from build123d import *

# Parameters (mm, degrees)
ESQUISSE1_R                            = 1.5
BOSS_EXTRU_1_DEPTH                     = 4
ESQUISSE2_R                            = 3.25
BOSS_EXTRU_2_DEPTH                     = 4
BOSS_EXTRU_3_START                     = -1
BOSS_EXTRU_3_DEPTH                     = 1
R_P_TITION_CIRCULAIRE6_COUNT           = 4
ESQUISSE5_R                            = 0.5
ENL_V_MAT_EXTRU_1_DEPTH                = 1
R_P_TITION_LIN_AIRE1_COUNT             = 3
R_P_TITION_LIN_AIRE1_PITCH             = 2
R_P_TITION_CIRCULAIRE7_COUNT           = 4
R_P_TITION_CIRCULAIRE7_COPY_1_SKETCH_R = 0.5
R_P_TITION_CIRCULAIRE7_COPY_1_DEPTH    = 1
R_P_TITION_CIRCULAIRE7_COPY_2_SKETCH_R = 0.5
R_P_TITION_CIRCULAIRE7_COPY_2_DEPTH    = 1
R_P_TITION_CIRCULAIRE7_COPY_3_SKETCH_R = 0.5
R_P_TITION_CIRCULAIRE7_COPY_3_DEPTH    = 1
R_P_TITION_CIRCULAIRE7_COPY_4_SKETCH_R = 0.5
R_P_TITION_CIRCULAIRE7_COPY_4_DEPTH    = 1
R_P_TITION_CIRCULAIRE7_COPY_5_SKETCH_R = 0.5
R_P_TITION_CIRCULAIRE7_COPY_5_DEPTH    = 1
R_P_TITION_CIRCULAIRE7_COPY_6_SKETCH_R = 0.5
R_P_TITION_CIRCULAIRE7_COPY_6_DEPTH    = 1
ESQUISSE6_R                            = 2.5
ENL_V_MAT_EXTRU_2_DEPTH                = 1
ESQUISSE7_R                            = 0.75
ENL_V_MAT_EXTRU_3_DEPTH                = 2


with BuildPart() as part:
    # Esquisse1 → Boss.-Extru.1 (new body)
    with BuildSketch(Plane(origin=(0, 0, 0), x_dir=(1, 0, 0), z_dir=(0, 1, 0))):
        with Locations(Location((0, 0, 0), (0, 0, 270))):
            Circle(ESQUISSE1_R)
    extrude(amount=BOSS_EXTRU_1_DEPTH)

    # Esquisse2 → Boss.-Extru.2 (add)
    with BuildSketch(Plane(origin=(0, 4, 0), x_dir=(1, 0, 0), z_dir=(0, 1, 0))):
        with Locations(Location((0, 0, 0), (0, 0, 270))):
            Circle(ESQUISSE2_R)
    extrude(amount=BOSS_EXTRU_2_DEPTH)

    # Esquisse3 → Boss.-Extru.3 (add)
    with BuildSketch(Plane(origin=(0, 8, 0), x_dir=(1, 0, 0), z_dir=(0, 1, 0)).offset(BOSS_EXTRU_3_START)):
        with BuildLine():
            ThreePointArc((-2, -8.5), (-1.25, -9.583333333), (0, -10))
            ThreePointArc((0, -10), (1.25, -9.583333333), (2, -8.5))
            Line((2, -8.5), (2, -2.561737691))
            ThreePointArc((2, -2.561737691), (0, -3.25), (-2, -2.561737691))
            Line((-2, -2.561737691), (-2, -8.5))
        make_face()
    boss_extru_3 = extrude(amount=BOSS_EXTRU_3_DEPTH)

    # Répétition circulaire6: Boss.-Extru.3 ×4 about axis
    r_p_tition_circulaire6_axis = Axis((0, 0, 0), (0, 1, 0))
    for i in range(1, R_P_TITION_CIRCULAIRE6_COUNT):
        add(boss_extru_3.rotate(r_p_tition_circulaire6_axis, i * 360 / R_P_TITION_CIRCULAIRE6_COUNT))

    # Esquisse5 → Enlèv. mat.-Extru.1 (cut)
    with BuildSketch(Plane(origin=(0, 8, 0), x_dir=(1, 0, 0), z_dir=(0, 1, 0))):
        with Locations(Location((0, -8.5, 0), (0, 0, 270))):
            Circle(ESQUISSE5_R)
    enl_v_mat_extru_1 = extrude(amount=-ENL_V_MAT_EXTRU_1_DEPTH, mode=Mode.SUBTRACT)

    # Répétition linéaire1: Enlèv. mat.-Extru.1 ×3
    with Locations(*[(0, 0, -i * R_P_TITION_LIN_AIRE1_PITCH) for i in range(1, R_P_TITION_LIN_AIRE1_COUNT)]):
        add(enl_v_mat_extru_1, mode=Mode.SUBTRACT)

    # Répétition circulaire7: Enlèv. mat.-Extru.1 ×4 about axis
    r_p_tition_circulaire7_axis = Axis((0, 0, 0), (0, 1, 0))
    for i in range(1, R_P_TITION_CIRCULAIRE7_COUNT):
        add(enl_v_mat_extru_1.rotate(r_p_tition_circulaire7_axis, i * 360 / R_P_TITION_CIRCULAIRE7_COUNT), mode=Mode.SUBTRACT)

    # Répétition circulaire7 copy 1 sketch → Répétition circulaire7 copy 1 (cut)
    with BuildSketch(Plane(origin=(-2, 8, 0), x_dir=(0, 0, -1), z_dir=(0, 1, 0))):
        with Locations(Location((0, -8.5, 0), (0, 0, 270))):
            Circle(R_P_TITION_CIRCULAIRE7_COPY_1_SKETCH_R)
    extrude(amount=-R_P_TITION_CIRCULAIRE7_COPY_1_DEPTH, mode=Mode.SUBTRACT)

    # Répétition circulaire7 copy 2 sketch → Répétition circulaire7 copy 2 (cut)
    with BuildSketch(Plane(origin=(0, 8, 2), x_dir=(-1, 0, 0), z_dir=(0, 1, 0))):
        with Locations(Location((0, -8.5, 0), (0, 0, 270))):
            Circle(R_P_TITION_CIRCULAIRE7_COPY_2_SKETCH_R)
    extrude(amount=-R_P_TITION_CIRCULAIRE7_COPY_2_DEPTH, mode=Mode.SUBTRACT)

    # Répétition circulaire7 copy 3 sketch → Répétition circulaire7 copy 3 (cut)
    with BuildSketch(Plane(origin=(2, 8, 0), x_dir=(0, 0, 1), z_dir=(0, 1, 0))):
        with Locations(Location((0, -8.5, 0), (0, 0, 270))):
            Circle(R_P_TITION_CIRCULAIRE7_COPY_3_SKETCH_R)
    extrude(amount=-R_P_TITION_CIRCULAIRE7_COPY_3_DEPTH, mode=Mode.SUBTRACT)

    # Répétition circulaire7 copy 4 sketch → Répétition circulaire7 copy 4 (cut)
    with BuildSketch(Plane(origin=(-4, 8, 0), x_dir=(0, 0, -1), z_dir=(0, 1, 0))):
        with Locations(Location((0, -8.5, 0), (0, 0, 270))):
            Circle(R_P_TITION_CIRCULAIRE7_COPY_4_SKETCH_R)
    extrude(amount=-R_P_TITION_CIRCULAIRE7_COPY_4_DEPTH, mode=Mode.SUBTRACT)

    # Répétition circulaire7 copy 5 sketch → Répétition circulaire7 copy 5 (cut)
    with BuildSketch(Plane(origin=(0, 8, 4), x_dir=(-1, 0, 0), z_dir=(0, 1, 0))):
        with Locations(Location((0, -8.5, 0), (0, 0, 270))):
            Circle(R_P_TITION_CIRCULAIRE7_COPY_5_SKETCH_R)
    extrude(amount=-R_P_TITION_CIRCULAIRE7_COPY_5_DEPTH, mode=Mode.SUBTRACT)

    # Répétition circulaire7 copy 6 sketch → Répétition circulaire7 copy 6 (cut)
    with BuildSketch(Plane(origin=(4, 8, 0), x_dir=(0, 0, 1), z_dir=(0, 1, 0))):
        with Locations(Location((0, -8.5, 0), (0, 0, 270))):
            Circle(R_P_TITION_CIRCULAIRE7_COPY_6_SKETCH_R)
    extrude(amount=-R_P_TITION_CIRCULAIRE7_COPY_6_DEPTH, mode=Mode.SUBTRACT)

    # Esquisse6 → Enlèv. mat.-Extru.2 (cut)
    with BuildSketch(Plane(origin=(0, 8, 0), x_dir=(1, 0, 0), z_dir=(0, 1, 0))):
        with Locations(Location((0, 0, 0), (0, 0, 270))):
            Circle(ESQUISSE6_R)
    extrude(amount=-ENL_V_MAT_EXTRU_2_DEPTH, mode=Mode.SUBTRACT)

    # Esquisse7 → Enlèv. mat.-Extru.3 (cut)
    with BuildSketch(Plane(origin=(0, 7, 0), x_dir=(1, 0, 0), z_dir=(0, 1, 0))):
        with Locations(Location((0, 0, 0), (0, 0, 270))):
            Circle(ESQUISSE7_R)
    extrude(amount=-ENL_V_MAT_EXTRU_3_DEPTH, mode=Mode.SUBTRACT)


solid = part.part
Here's how the part is built. I have some questions about the finished solid (model axes, mm). A direction names the side the tool comes from. Coordinates: 2 decimals unless noted, no trailing zeros. Write each loop counter-clockwise with the first axis right and the second up, starting at its lowest first coordinate (ties: lowest second). Pieces come first, ordered by that corner, then holes.
1) I'm going to push flat-ended pins straight in: pin 1 (5 mm diameter, centred on x = -4.5, z = 3.5, fed in from -Y); pin 2 (0.8 mm diameter, centred on y = 7.5, z = 6.5, fed in from -X); pin 3 (2 mm diameter, centred on x = 4, z = 2.5, fed in from +Y); pin 4 (2 mm diameter, centred on x = 0, z = 7.5, fed in from -Y). Where does each tip first touch, or does it pass through?
Filled in:
pin 1: stops at y = 4
pin 2: stops at x = -2
pin 3: stops at y = 8
pin 4: stops at y = 7
2) If we section it at B-B (z = -6.5): List the corners of the cut face in (x, y) for me.
Filled in:
outline: (-2, 7) - (-0.5, 7) - (-0.5, 8) - (-2, 8) - close; (0.5, 7) - (2, 7) - (2, 8) - (0.5, 8) - close
3) Which directions (+Z, -Z, +X, -X, +Y, -Y) give clear straight access to the entire face, cutting with the end or side of a thin tool? Please do faces 5 (the face through (1.5, 4, 0.7)), 6 (the face through (0, 0, 0)), 7 (the face through (2, 7.5, 5.6)).
Filled in:
face 5: -Y
face 6: +Z, -Z, +X, -X, -Y
face 7: +Z, +X, +Y, -Y
4) Thinking about a two-plate mould opening in X: for faces 1 (the face through (-0.4, 7, -7.1)), 2 (the face through (0.45, 1.97, 1.43)), 3 (the face through (-2, 7.5, 5.5)), 4 (the face through (0.192, 7.507, -6.962)), which applies, +X half, -X half, draft (parallel to the pull), parting line (faces both ways), or undercut?
Filled in:
face 1: draft
face 2: parting line
face 3: -X half
face 4: undercut
5) If we section it at A-A (x = 6.5): List the corners of the cut face in (y, z) for me.
Filled in:
outline: (7, -2) - (8, -2) - (8, -0.5) - (7, -0.5) - close; (7, 0.5) - (8, 0.5) - (8, 2) - (7, 2) - close
6) If I drill on line 1 (X direction, y = 7.4, z = -4.5); line 2 (Y direction, x = 1.25, z = 7.25), over which ranges is the centre line in solid material (lowest first)?
Filled in:
line 1: x = -2 to -0.5, 0.5 to 2
line 2: y = 7 to 8
7) If we section it at C-C (x = 1): List the corners of the cut face in (y, z) for me, plus the area to 3 significant figures.
Filled in:
outline: (0, -1.12) - (4, -1.12) - (4, -3.09) - (7, -3.09) - (7, -9.74) - (8, -9.74) - (8, -2.29) - (7, -2.29) - (7, 2.29) - (8, 2.29) - (8, 9.74) - (7, 9.74) - (7, 3.09) - (4, 3.09) - (4, 1.12) - (0, 1.12) - close
area: 42.4 mm2
8) If we section it at D-D (y = 6.25): List the corners of the cut face in (x, z) for me, plus the area to 3 significant figures.
Filled in:
outline: circle Ø6.5 at (0, 0); hole circle Ø1.5 at (0, 0)
area: 31.4 mm2
